from build123d import *

# Parameters (mm, degrees)
ESBO_O1_R                = 3
ESBO_O1_R_2              = 1.6
ESBO_O1_W                = 15
ESBO_O1_H                = 3
ESBO_O1_W_2              = 42
ESBO_O1_H_2              = 21
ESBO_O1_R_3              = 9.5
ESBO_O1_H_3              = 6
RESSALTO_EXTRUS_O1_DEPTH = 6
FILETE1_R                = 5
ESBO_O2_W                = 15
ESBO_O2_H                = 1.3
ESBO_O2_W_2              = 5
ESBO_O2_H_2              = 3
CORTE_EXTRUS_O1_DEPTH    = 183.363523005
ESBO_O3_W                = 15
ESBO_O3_H                = 1.3
RESSALTO_EXTRUS_O2_DEPTH = 6


with BuildPart() as part:
    # Esboço1 → Ressalto-extrusão1 (new body)
    with BuildSketch(Plane.XZ.offset(6)):
        with BuildLine():
            ThreePointArc((28.221137594, -123.946334359), (26.32780231, -130.898758331), (30.793557575, -136.55366306))
            Line((30.793557575, -136.55366306), (52.89462836, -146.829127406))
            ThreePointArc((52.89462836, -146.829127406), (53.923154275, -147.177291613), (55.00259, -147.2952))
            Line((55.00259, -147.2952), (102.35259, -147.2952))
            ThreePointArc((102.35259, -147.2952), (105.888123906, -145.830733906), (107.35259, -142.2952))
            Line((107.35259, -142.2952), (107.35259, -122.2))
            ThreePointArc((107.35259, -122.2), (105.888123906, -118.664466094), (102.35259, -117.2))
            Line((102.35259, -117.2), (88.05, -117.2))
            ThreePointArc((88.05, -117.2), (84.514466094, -115.735533906), (83.05, -112.2))
            Line((83.05, -112.2), (83.05, -110.8795617))
            Line((83.05, -110.8795617), (96.038503575, -100.173097388))
            ThreePointArc((96.038503575, -100.173097388), (98.95, -94), (96.038503575, -87.826902612))
            Line((96.038503575, -87.826902612), (88.137508625, -81.314087647))
            Line((88.137508625, -81.314087647), (103.678862406, -64.053665641))
            ThreePointArc((103.678862406, -64.053665641), (103.086748653, -52.755462186), (91.788545198, -53.347575939))
            Line((91.788545198, -53.347575939), (85.037246259, -60.845653032))
            ThreePointArc((85.037246259, -60.845653032), (83.355205347, -62.067727288), (81.321522132, -62.5))
            Line((81.321522132, -62.5), (53.85, -62.5))
            ThreePointArc((53.85, -62.5), (50.314466094, -63.964466094), (48.85, -67.5))
            Line((48.85, -67.5), (48.85, -77.1204383))
            Line((48.85, -77.1204383), (35.861496425, -87.826902612))
            ThreePointArc((35.861496425, -87.826902612), (32.95, -94), (35.861496425, -100.173097388))
            Line((35.861496425, -100.173097388), (43.762491375, -106.685912353))
            Line((43.762491375, -106.685912353), (28.221137594, -123.946334359))
        make_face()
        with Locations(Location((34.166296198, -129.29937921, 0), (0, 0, 270))):
            Circle(ESBO_O1_R, mode=Mode.SUBTRACT)
        with Locations(Location((51.25259, -136.7952, 0), (0, 0, 270))):
            Circle(ESBO_O1_R_2, mode=Mode.SUBTRACT)
        with Locations(Location((51.25259, -126.7952, 0), (0, 0, 270))):
            Circle(ESBO_O1_R_2, mode=Mode.SUBTRACT)
        with Locations((65.95, -115.7)):
            Rectangle(ESBO_O1_W, ESBO_O1_H, mode=Mode.SUBTRACT)
        with Locations((65.95, -106.5)):
            Rectangle(ESBO_O1_W, ESBO_O1_H, mode=Mode.SUBTRACT)
        with Locations((76.00259, -131.7952)):
            Rectangle(ESBO_O1_W_2, ESBO_O1_H_2, mode=Mode.SUBTRACT)
        with Locations(Location((100.75259, -136.7952, 0), (0, 0, 270))):
            Circle(ESBO_O1_R_2, mode=Mode.SUBTRACT)
        with Locations(Location((100.75259, -126.7952, 0), (0, 0, 270))):
            Circle(ESBO_O1_R_2, mode=Mode.SUBTRACT)
        with Locations(Location((65.95, -94, 0), (0, 0, 270))):
            Circle(ESBO_O1_R_3, mode=Mode.SUBTRACT)
        with Locations((65.95, -70.5)):
            Rectangle(ESBO_O1_W, ESBO_O1_H_3, mode=Mode.SUBTRACT)
        with Locations(Location((97.733703802, -58.70062079, 0), (0, 0, 270))):
            Circle(ESBO_O1_R, mode=Mode.SUBTRACT)
        with Locations(Location((40.95, -94, 0), (0, 0, 270))):
            Circle(ESBO_O1_R_2, mode=Mode.SUBTRACT)
        with Locations(Location((90.95, -94, 0), (0, 0, 270))):
            Circle(ESBO_O1_R_2, mode=Mode.SUBTRACT)
    extrude(amount=-RESSALTO_EXTRUS_O1_DEPTH)

    # Filete1
    # the kernel refuses this fillet: 5 mm, written as the material it adds along each edge
    with BuildSketch(Plane(origin=(83.05, -6, -110.8795617), x_dir=(0, 0, -1), z_dir=(0, 1, 0))) as filete1_piece_1:
        with BuildLine():
            CenterArc((2.468290902, -4.866460151), FILETE1_R, 103.271787815, 37.229346276)
            Line((-1.389894966, -1.686145417), (-1.467058683, -1.622539122))
            Line((-1.467058683, -1.622539122), (-0.077163717, 0.063606295))
            Line((-0.077163717, 0.063606295), (0, 0.1))
            ThreePointArc((0, 0.1), (0.66021915, 0.1), (1.297481248, 0.097329203))
            Line((1.297481248, 0.097329203), (1.3204383, 0))
        make_face()
    extrude(amount=6)
    with BuildSketch(Plane(origin=(88.137508625, -6, -81.314087647), x_dir=(0.7716371735307594, 0, -0.6360629469049904), z_dir=(0, 1, 0))) as filete1_piece_2:
        with BuildLine():
            CenterArc((FILETE1_R * 1.04463432468, -FILETE1_R), FILETE1_R, 90, 92.501134091)
            Line((FILETE1_R * 0.045586966675, -FILETE1_R * 1.04363916214), (FILETE1_R * 0.025606019515, -FILETE1_R * 1.04451194539))
            Line((FILETE1_R * 0.025606019515, -FILETE1_R * 1.04451194539), (-FILETE1_R * 0.0208926864935, FILETE1_R * 0.02))
            Line((-FILETE1_R * 0.0208926864935, FILETE1_R * 0.02), (FILETE1_R * 1.04463432468, FILETE1_R * 0.02))
            Line((FILETE1_R * 1.04463432468, FILETE1_R * 0.02), (FILETE1_R * 1.04463432468, 0))
        make_face()
    extrude(amount=6)
    with BuildSketch(Plane(origin=(48.85, -6, -77.1204383), x_dir=(0, 0, 1), z_dir=(0, 1, 0))) as filete1_piece_3:
        with BuildLine():
            CenterArc((FILETE1_R * 0.471642717043, -FILETE1_R), FILETE1_R, 90, 50.501134091)
            Line((-FILETE1_R * 0.299994456488, -FILETE1_R * 0.363937053095), (-FILETE1_R * 0.315427199959, -FILETE1_R * 0.351215794157))
            Line((-FILETE1_R * 0.315427199959, -FILETE1_R * 0.351215794157), (-FILETE1_R * 0.00943285434085, FILETE1_R * 0.02))
            Line((-FILETE1_R * 0.00943285434085, FILETE1_R * 0.02), (FILETE1_R * 0.471642717043, FILETE1_R * 0.02))
            Line((FILETE1_R * 0.471642717043, FILETE1_R * 0.02), (FILETE1_R * 0.471642717043, 0))
        make_face()
    extrude(amount=6)
    with BuildSketch(Plane(origin=(43.762491375, -6, -106.685912353), x_dir=(-0.6691306063588565, 0, -0.7431448254773958), z_dir=(0, 1, 0))) as filete1_piece_4:
        with BuildLine():
            CenterArc((FILETE1_R * 1.04463432468, FILETE1_R), FILETE1_R, 177.498865909, 92.501134091)
            Line((FILETE1_R * 0.0455869666753, FILETE1_R * 1.04363916214), (FILETE1_R * 0.0256060195153, FILETE1_R * 1.04451194539))
            Line((FILETE1_R * 0.0256060195153, FILETE1_R * 1.04451194539), (-FILETE1_R * 0.0208926864935, -FILETE1_R * 0.02))
            Line((-FILETE1_R * 0.0208926864935, -FILETE1_R * 0.02), (FILETE1_R * 1.04463432468, -FILETE1_R * 0.02))
            Line((FILETE1_R * 1.04463432468, -FILETE1_R * 0.02), (FILETE1_R * 1.04463432468, 0))
        make_face()
    extrude(amount=6)

    # Esboço2 → Corte-extrusão1 (cut, through all)
    with BuildSketch(Plane.XZ.offset(6)):
        with Locations((65.95, -104.35)):
            Rectangle(ESBO_O2_W, ESBO_O2_H)
        with Locations((52.50259, -131.7952)):
            Rectangle(ESBO_O2_W_2, ESBO_O2_H_2)
        with Locations((99.50259, -131.7952)):
            Rectangle(ESBO_O2_W_2, ESBO_O2_H_2)
    extrude(amount=-CORTE_EXTRUS_O1_DEPTH, mode=Mode.SUBTRACT)

    # Esboço3 → Ressalto-extrusão2 (add)
    with BuildSketch(Plane.XZ.offset(6)):
        with Locations((65.95, -107.35)):
            Rectangle(ESBO_O3_W, ESBO_O3_H)
    extrude(amount=-RESSALTO_EXTRUS_O2_DEPTH)


solid = part.part
Input: part model. Units: mm. Frame: model coordinates. A direction names the side the tool comes from. Coordinates: 2 decimals unless noted, no trailing zeros. Order: outer loops, then holes, each group sorted by start corner. A loop starts at its lowest first (then second) coordinate and runs counter-clockwise, first axis right, second up. Notation, with made-up numbers: M 47.25,82 L 51.25,82 A36 ccw 51.25,118 Z; hole C 86.5,43.5 d1. An arc over 180 degrees is marked long. Answer as CSV lines item,"result".
1. Section D-D (z = -80). Return the cut outline in (x, y), then the cut area to 3 significant figures.
Reported:
outline,"M 45.36,-6 L 90.41,-6 L 90.41,0 L 45.36,0 Z"
area,"270 mm2"
2. Pull-direction query (Z, two-part tool) for faces 3 (the flat face through (37.77, -3.042, -101.746)), 4 (the cylindrical face through (32.95, -3.04, -93.9)), 5 (the flat face through (107.353, -3, -132)); classes: released by +Z, released by -Z, zero draft, split by the parting line, or undercut.
Reported:
face 3,"undercut"
face 4,"undercut"
face 5,"zero draft"
3. Section C-C (y = -1.7). State how many separate pieces and enclosed holes the cut face has, then the cut area to 3 significant figures.
Reported:
separate pieces,"1"
enclosed holes,"13"
area,"3,780 mm2"
4. Access query for faces 1 (the flat face through (76, -3, -142.295)), 2 (the flat face through (90.308, -3.042, -104.897)). Directions: +Z, -Z, +X, -X, +Y, -Y. A direction counts if a zero-diameter tool reaches every point of the face in a straight line with its end or side. Return the directions, or none.
Reported:
face 1,"+Y, -Y"
face 2,"+X, +Y, -Y"
5. Material intervals for line 1 (Z direction, x = 70, y = -3.75); line 2 (Z direction, x = 90, y = -3.55); line 3 (Z direction, x = 74.5, y = -1.15), sorted ascending. Write a range as from..to.
Reported:
line 1,"-147.3..-142.3, -121.3..-117.2, -114.2..-106.7, -103.7..-102.59, -85.41..-73.5, -67.5..-62.5"
line 2,"-147.3..-142.3, -121.3..-117.2, -105.15..-95.29, -92.71..-55.33"
line 3,"-147.3..-142.3, -121.3..-98.14, -89.86..-62.5"
6. Section B-B (x = 71). Return the cut outline in (y, z).
Reported:
outline,"M -6,-147.3 L 0,-147.3 L 0,-142.3 L -6,-142.3 Z; M -6,-121.3 L 0,-121.3 L 0,-117.2 L -6,-117.2 Z; M -6,-114.2 L 0,-114.2 L 0,-106.7 L -6,-106.7 Z; M -6,-103.7 L 0,-103.7 L 0,-102.05 L -6,-102.05 Z; M -6,-85.95 L 0,-85.95 L 0,-73.5 L -6,-73.5 Z; M -6,-67.5 L 0,-67.5 L 0,-62.5 L -6,-62.5 Z"
7. First-contact query: P1, Ø1.5, axis at y = -2, z = -113, coming from the +X side; P2, Ø1.5, axis at y = -4, z = -76, coming from the +X side; P3, Ø2, axis at y = -4.5, z = -98.5, coming from the +X side; P4, Ø1.9, axis at x = 90.95, z = -94, coming from the -Y side. Flat tips, straight axial feed; report the tip coordinate or a pass-through.
Reported:
P1,"x = 83.3"
P2,"x = 93.6"
P3,"x = 98.14"
P4,"through"
8. Section A-A (z = -94). Return the cut outline in (x, y), then the cut area to 3 significant figures.
Reported:
outline,"M 32.95,-6 L 39.35,-6 L 39.35,0 L 32.95,0 Z; M 42.55,-6 L 56.45,-6 L 56.45,0 L 42.55,0 Z; M 75.45,-6 L 89.35,-6 L 89.35,0 L 75.45,0 Z; M 92.55,-6 L 98.95,-6 L 98.95,0 L 92.55,0 Z"
area,"244 mm2"
